Check sheet for the modelled part. Datum: model origin and axes. Units: mm. Face numbers are marked on the shaded views. Round coordinates to 2 decimals unless told otherwise and drop trailing zeros. Loops run counter-clockwise (first coordinate to the right, second up) from the corner with the lowest first, then second, coordinate; pieces in that order, holes last. Notation, with made-up numbers: M 44,-17.75 L 90,-17.75 A30 ccw 90,16.25 Z; hole C -7,-7 d7. An arc over 180 degrees is marked long. Write item = value, one per line. Start each with the question number.
(1) Cross-section at D-D on x = 0. Record the boundary of the cut face in (y, z).
(2) Cross-section at B-B on z = 18. Record the boundary of the cut face in (x, y).
(3) Mould release check, pull along X, two halves, no side actions. Record for the marked faces 1, 2, 3 and 4: pulls with the +X half, pulls with the -X half, needs draft (parallel to the pull), parting line crosses it, or undercut.
(4) Go/stop test with a flat-tipped pin: P1, Ø6.5, axis at y = 6, z = 0, coming from the +X side. Record where the tip stops, or that it passes through.
(5) Cross-section at C-C on y = 9.75. Record the boundary of the cut face in (x, z), plus the area to 3 significant figures.
(6) Cross-section at A-A on y = 6. Record the boundary of the cut face in (x, z).
(7) Scan lines: L1, parallel to Z at x = 0, y = 5; L2, parallel to Z at x = 8.5, y = 6; L3, parallel to Z at x = 1, y = 3.5. Record each from-to range of solid material in increasing order. Write a range as from..to.
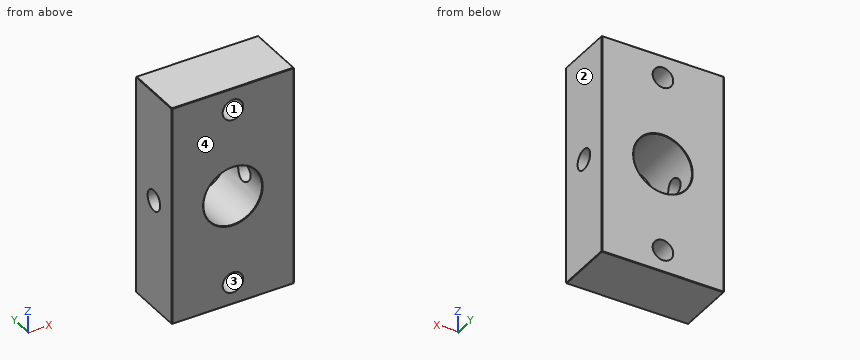
from build123d import *

# Parameters (mm, degrees)
SKETCH1_W           = 25
SKETCH1_H           = 45
SKETCH1_R           = 6
BOSS_EXTRUDE1_DEPTH = 12
M5_TAPPED_HOLE2_D   = 4.2
M5_TAPPED_HOLE3_D   = 4.2
CHAMFER1_SIZE       = 0.1


with BuildPart() as part:
    # Sketch1 → Boss-Extrude1 (new body)
    with BuildSketch(Plane(origin=(0, 0, 0), x_dir=(1, 0, 0), z_dir=(0, 1, 0))):
        Rectangle(SKETCH1_W, SKETCH1_H)
        Circle(SKETCH1_R, mode=Mode.SUBTRACT)
    extrude(amount=BOSS_EXTRUDE1_DEPTH)

    # M5 Tapped Hole2 (through all)
    with Locations(Plane(origin=(0, 12, 0), x_dir=(1, 0, 0), z_dir=(0, 1, 0))):
        with Locations((0, 18), (0, -18)):
            Hole(M5_TAPPED_HOLE2_D / 2)

    # M5 Tapped Hole3 (through all)
    with Locations(Plane.ZY.offset(12.5)):
        with Locations((0, 6)):
            Hole(M5_TAPPED_HOLE3_D / 2)

    # Chamfer1
    chamfer1_edges = [part.edges().sort_by_distance(p)[0] for p in [
        (-6, 0, 0),
        (-6, 12, 0),
        (-12.5, 12, 0),
        (0, 12, 22.5),
        (12.5, 12, 0),
        (0, 0, 22.5),
        (-12.5, 0, 0),
        (0, 0, -22.5),
        (12.5, 0, 0),
        (12.5, 6, 22.5),
        (-12.5, 6, 22.5),
        (-12.5, 6, -22.5),
        (12.5, 6, -22.5),
        (0, 12, -22.5),
    ]]
    chamfer(chamfer1_edges, length=CHAMFER1_SIZE)


solid = part.part
Result:
q1.outline = M 0,-22.4 L 0.1,-22.5 L 11.9,-22.5 L 12,-22.4 L 12,-20.1 L 0,-20.1 Z; M 0,-15.9 L 12,-15.9 L 12,-6.1 L 11.9,-6 L 0.1,-6 L 0,-6.1 Z; M 0,6.1 L 0.1,6 L 11.9,6 L 12,6.1 L 12,15.9 L 0,15.9 Z; M 0,20.1 L 12,20.1 L 12,22.4 L 11.9,22.5 L 0.1,22.5 L 0,22.4 Z
q2.outline = M -12.5,0.1 L -12.4,0 L -2.1,0 L -2.1,12 L -12.4,12 L -12.5,11.9 Z; M 2.1,0 L 12.4,0 L 12.5,0.1 L 12.5,11.9 L 12.4,12 L 2.1,12 Z
q3.face_1 = undercut
q3.face_2 = pulls with the +X half
q3.face_3 = undercut
q3.face_4 = needs draft
q4.P1 = 12.5
q5.outline = M -12.5,-22.4 L -12.4,-22.5 L 12.4,-22.5 L 12.5,-22.4 L 12.5,22.4 L 12.4,22.5 L -12.4,22.5 L -12.5,22.4 Z; hole C 0,0 d12; hole C 0,-18 d4.2; hole C 0,18 d4.2
q5.area = 984 mm^2
q6.outline = M -12.5,-22.4 L -12.4,-22.5 L 12.4,-22.5 L 12.5,-22.4 L 12.5,-2.1 L 5.62,-2.1 A6 cw -5.62,-2.1 L -12.5,-2.1 Z; M -12.5,2.1 L -5.62,2.1 A6 cw 5.62,2.1 L 12.5,2.1 L 12.5,22.4 L 12.4,22.5 L -12.4,22.5 L -12.5,22.4 Z; hole C 0,-18 d4.2; hole C 0,18 d4.2
q7.L1 = -22.5..-20.1, -15.9..-6, 6..15.9, 20.1..22.5
q7.L2 = -22.5..-2.1, 2.1..22.5
q7.L3 = -22.5..-19.85, -16.15..-5.92, 5.92..16.15, 19.85..22.5
